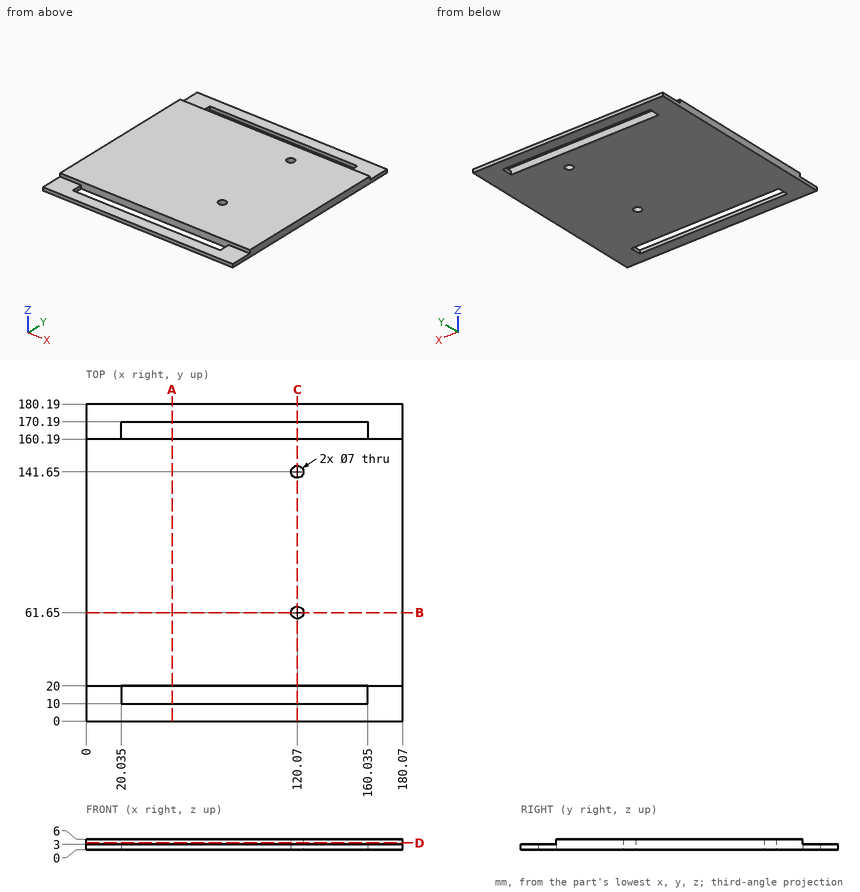
Can you work these out from the drawing? Everything is in mm from the part's minimum corner. Round coordinates to 2 decimals unless told otherwise and drop trailing zeros. Order: outer loops, then holes, each group sorted by start corner. A loop starts at its lowest first (then second) coordinate and runs counter-clockwise, first axis right, second up. Notation, with made-up numbers: M 13,70.5 L 47,70.5 A18 ccw 47,105.5 Z; hole C 88.25,52 d8. An arc over 180 degrees is marked long. One line per question, with ' | ' between items.
1) For pin 1 Ø10 at (x, y) = (125, 168) entering from +Z, with a flat end and sliding along its axis, tell me the tip position at first contact or that it passes through.
Working result:
pin 1: z = 3
2) I want a section at D-D, the plane z = 3.9. Write out the boundary of the cut face in (x, y).
Working result:
outline: M 0,20 L 180.07,20 L 180.07,160.19 L 0,160.19 Z; hole C 120.07,61.65 d7; hole C 120.07,141.65 d7
3) I want a section at A-A, the plane x = 49. Write out the boundary of the cut face in (y, z).
Working result:
outline: M 0,0 L 10,0 L 10,3 L 0,3 Z; M 20,0 L 160.19,0 L 160.19,6 L 20,6 Z; M 170.19,0 L 180.19,0 L 180.19,3 L 170.19,3 Z
4) I want a section at B-B, the plane y = 61.65. Write out the boundary of the cut face in (x, z), then the cut area to 3 significant figures.
Working result:
outline: M 0,0 L 116.57,0 L 116.57,6 L 0,6 Z; M 123.57,0 L 180.07,0 L 180.07,6 L 123.57,6 Z | area: 1,040 mm²
5) I need wall thicknesses on line 1 along Y through (x, z) = (154.5, 1.95); line 2 along Y through (x, z) = (120.07, 3.1); line 3 along Y through (x, z) = (120.07, 2.15). Which ranges of each line are inside material? Lowest first, please.
Working result:
line 1: 0 to 10, 20 to 160.19, 170.19 to 180.19 | line 2: 20 to 58.15, 65.15 to 138.15, 145.15 to 160.19 | line 3: 0 to 10, 20 to 58.15, 65.15 to 138.15, 145.15 to 160.19, 170.19 to 180.19
6) I want a section at C-C, the plane x = 120.07. Write out the boundary of the cut face in (y, z).
Working result:
outline: M 0,0 L 10,0 L 10,3 L 0,3 Z; M 20,0 L 58.15,0 L 58.15,6 L 20,6 Z; M 65.15,0 L 138.15,0 L 138.15,6 L 65.15,6 Z; M 145.15,0 L 160.19,0 L 160.19,6 L 145.15,6 Z; M 170.19,0 L 180.19,0 L 180.19,3 L 170.19,3 Z
